Source: CAD feature listing. Evaluate the final solid. Frame: model axes, mm. Give positions to 0.01 mm unless a question says otherwise; leave off trailing zeros. Write each loop counter-clockwise with the first axis right and the second up, starting at its lowest first coordinate (ties: lowest second). Pieces come first, ordered by that corner, then holes. Notation, with made-up numbers: M 53.25,-29 L 76.25,-29 A13 ccw 76.25,-23 Z; hole C 69.25,-30 d3. An arc over 180 degrees is marked long. Use CSV: the item, a comma, the result in double quotes. Start each with the question number.
from build123d import *

# Parameters (mm, degrees)
F0_W        = 120
F0_H        = 28
F1_DEPTH    = 462.5
F2_SIZE2    = 115.882643
F2_SIZE     = 119.99999
F3_T1_DEPTH = 343.6641668027


# Not quite as in the source:
# - a fillet or chamfer that OpenCascade refuses, or shapes differently, is made with other operations: its cross-section is extruded or revolved along the edge and cut away or added
# - a fillet or chamfer is up to 0.001 mm smaller than in the source, because OpenCascade refuses the exact size


with BuildPart() as f1:
    # F0 (on Front) → F1 (new body, symmetric)
    with BuildSketch(Plane.XZ):
        Rectangle(F0_W, F0_H)
    extrude(amount=F1_DEPTH, both=True)

    # F2 (size 120 and 115.8826529768 in the source; OpenCascade refuses exactly that, so slightly less here)
    f2_edges = [f1.edges().sort_by_distance(p)[0] for p in [
        (60, -462.5, 0),
    ]]
    f2_side = f1.faces().sort_by_distance((0, -462.5, 0))[0]
    chamfer(f2_edges, length=F2_SIZE, length2=F2_SIZE2, reference=f2_side)

    # F3: chamfer of 6 x 34.0276909177 on 2 edges, made by hand

    # F3_s2 → F3_t1 (cut)
    with BuildSketch(Plane(origin=(-325.7617702656, -314.5844839382, 0), x_dir=(0, 0, 1), z_dir=(0.7193398013, 0.6946583695, 0))):
        Polygon((-14, 285.0151628785), (20.0276909177, 291.0151628785), (-14, 291.0151628785), align=None)
    extrude(amount=F3_T1_DEPTH, mode=Mode.SUBTRACT)


solid = f1.part
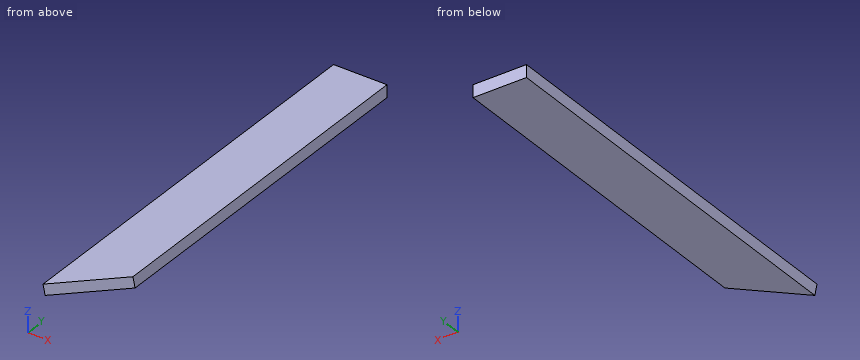
1. First-contact query: pin 1 (1 mm diameter, centred on x = -36, z = -4, fed in from -Y); pin 2 (10 mm diameter, centred on x = 10.5, z = 11, fed in from -Y). Flat tips, straight axial feed; report the tip coordinate or a pass-through.
2. Section A-A on z = 9.75. Return loops of the section in (x, y).
3. Line query: probe 1 along Y at (x, z) = (2, -0.25); probe 2 along X at (y, z) = (-410.5, 5); probe 3 along Y at (x, z) = (13, -1). Output: solid intervals per line, ascending.
4. Section B-B on x = -14. Return loops of the section in (y, z).
Resolved:
1,pin 1,"stops at y = -433.93"
1,pin 2,"stops at y = -397.19"
2,outline,"M -60,-459.98 L 60,-344.1 L 60,462.5 L -60,462.5 Z"
3,probe 1,"y = -397.66 to 462.5"
3,probe 2,"x = -60 to -9.97"
3,probe 3,"y = -386.85 to 462.5"
4,outline,"M -416.6,14 L -409.74,-14 L 462.5,-14 L 462.5,14 Z"
